Can you work these out from the drawing? Everything is in mm from the part's minimum corner. Round coordinates to 2 decimals unless told otherwise and drop trailing zeros. Write each loop counter-clockwise with the first axis right and the second up, starting at its lowest first coordinate (ties: lowest second). Pieces come first, ordered by that corner, then holes.
Q1. I'm going to push a flat-ended pin straight in: pin 1 Ø2.5 at (x, y) = (6, 12) entering from -Z. Where does the tip first touch, or does it pass through?
Q2. If we section it at D-D (y = 8.25): Please give me the cut outline in (x, z), plus the area to 3 significant figures.
Q3. If we section it at B-B (y = 12): Please give me the cut outline in (x, z), plus the area to 3 significant figures.
Q4. If we section it at C-C (z = 14): Please give me the cut outline in (x, y).
Q5. If we section it at A-A (x = 6): Please give me the cut outline in (y, z).
Q6. Please list where these lines run through material, in increasing order: line 1 along Z through (x, y) = (9, 5); line 2 along Y through (x, z) = (6, 10); line 3 along X through (y, z) = (5.5, 1.75).
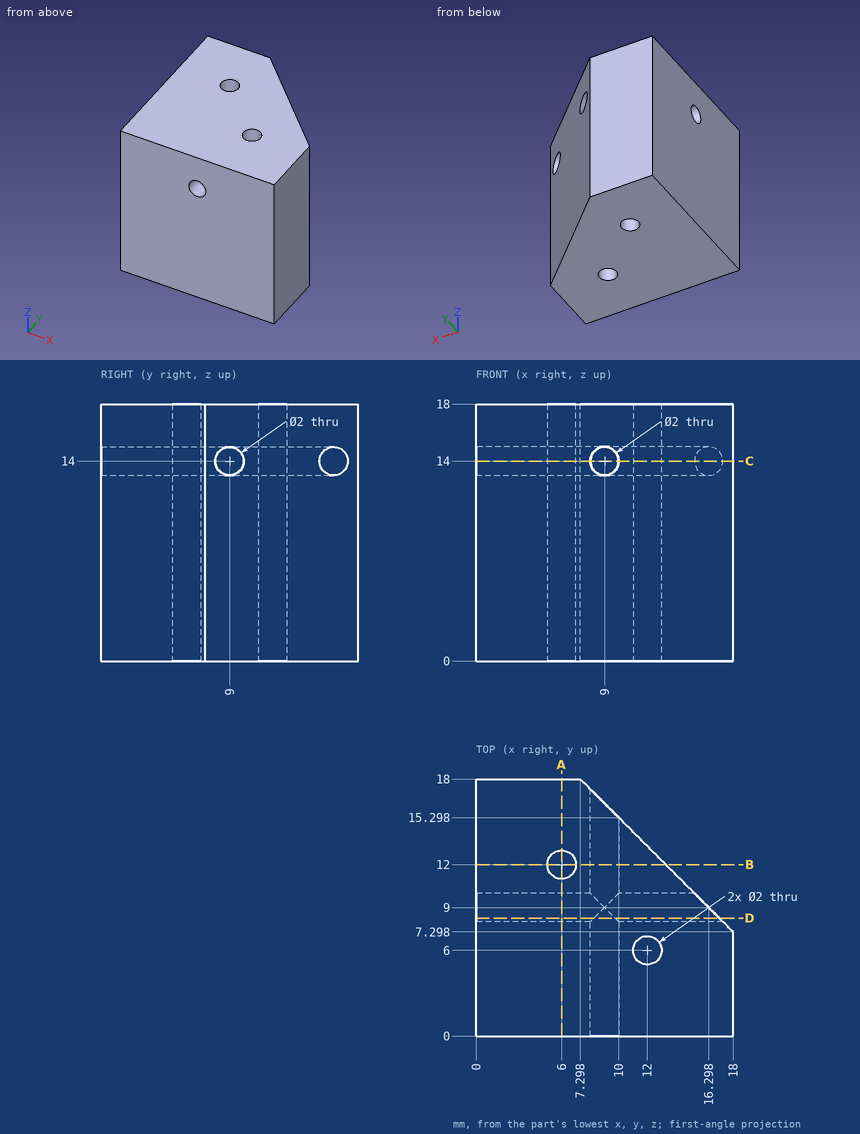
A:
1. pin 1: stops at z = 0
2. outline: (0, 0) - (17.05, 0) - (17.05, 13.34) - (9.75, 13.34) arc R1 cw to (8.25, 13.34) - (0, 13.34) - close; (0, 14.66) - (8.25, 14.66) arc R1 cw to (9.75, 14.66) - (17.05, 14.66) - (17.05, 18) - (0, 18) - close
2. area: 284 mm2
3. outline: (0, 0) - (5, 0) - (5, 18) - (0, 18) - close; (7, 0) - (13.3, 0) - (13.3, 18) - (7, 18) - close; hole circle Ø2 at (9, 14)
3. area: 200 mm2
4. outline: (0, 0) - (8, 0) - (8, 8) - (0, 8) - close; (0, 10) - (8, 10) - (8, 17.3) - (7.3, 18) - (0, 18) - close; (10, 0) - (18, 0) - (18, 7.3) - (17.3, 8) - (10, 8) - close; (10, 10) - (15.3, 10) - (10, 15.3) - close; hole circle Ø2 at (6, 12); hole circle Ø2 at (12, 6)
5. outline: (0, 0) - (11, 0) - (11, 18) - (0, 18) - close; (13, 0) - (18, 0) - (18, 18) - (13, 18) - close; hole circle Ø2 at (9, 14)
6. line 1: z = 0 to 13, 15 to 18
6. line 2: y = 0 to 11, 13 to 18
6. line 3: x = 0 to 11.13, 12.87 to 18
